```python
from build123d import *

# Parameters (mm, degrees)
SKETCH_W          = 64.5
SKETCH_H          = 46.5
PAD_DEPTH         = 25
SKETCH001_W       = 61
SKETCH001_H       = 42.5
POCKET_DEPTH      = 21
SKETCH002_R       = 2
POCKET001_DEPTH   = 4
POCKET002_DEPTH   = 2
POCKET003_DEPTH   = 2
SKETCH005_R       = 2
POCKET004_DEPTH   = 2
PAD001_DEPTH      = 10
PAD001_DEPTH_BACK = 2
PAD002_DEPTH      = 1
SKETCH008_R       = 5.5
PAD003_DEPTH      = 4
SKETCH009_W       = 5
SKETCH009_H       = 5
POCKET005_DEPTH   = 49.501
SKETCH010_W       = 5
SKETCH010_H       = 5
POCKET006_DEPTH   = 26.7259364864
SKETCH011_W       = 3
SKETCH011_H       = 6
SKETCH011_H_2     = 4
PAD004_DEPTH      = 2
POCKET007_DEPTH   = 5


with BuildPart() as part:
    # Sketch → Pad (new body)
    with BuildSketch(Plane.XZ):
        Rectangle(SKETCH_W, SKETCH_H)
    extrude(amount=PAD_DEPTH)

    # Sketch001 (on Face6 of Pad) → Pocket (cut)
    with BuildSketch(Plane.XZ.offset(25)):
        Rectangle(SKETCH001_W, SKETCH001_H)
    extrude(amount=-POCKET_DEPTH, mode=Mode.SUBTRACT)

    # Sketch002 (on Face11 of Pocket) → Pocket001 (cut)
    with BuildSketch(Plane.XZ.offset(4)):
        with Locations((24.5, 16.25)):
            Circle(SKETCH002_R)
    extrude(amount=-POCKET001_DEPTH, mode=Mode.SUBTRACT)

    # Sketch003 (on Face3 of Pocket001) → Pocket002 (cut)
    with BuildSketch(Plane(origin=(32.25, 0, 0), x_dir=(0, 0, 1), z_dir=(1, 0, 0))):
        with BuildLine():
            ThreePointArc((-7.25, 18.5), (-11.25, 14.5), (-7.25, 10.5))
            Line((-7.25, 10.5), (2.75, 10.5))
            ThreePointArc((2.75, 10.5), (6.75, 14.5), (2.75, 18.5))
            Line((-7.25, 18.5), (2.75, 18.5))
        make_face()
    extrude(amount=-POCKET002_DEPTH, mode=Mode.SUBTRACT)

    # Sketch004 (on Face1 of Pocket002) → Pocket003 (cut)
    with BuildSketch(Plane(origin=(0, 0, 23.25), x_dir=(-1, 0, 0), z_dir=(0, 0, 1))):
        with BuildLine():
            ThreePointArc((8.5, 21.5), (1, 14), (8.5, 6.5))
            Line((8.5, 6.5), (15.5, 6.5))
            ThreePointArc((15.5, 6.5), (23, 14), (15.5, 21.5))
            Line((8.5, 21.5), (15.5, 21.5))
        make_face()
    extrude(amount=-POCKET003_DEPTH, mode=Mode.SUBTRACT)

    # Sketch005 (on Face10 of Pocket003) → Pocket004 (cut)
    with BuildSketch(Plane(origin=(0, 0, -23.25), x_dir=(1, 0, 0), z_dir=(0, 0, -1))):
        with Locations((-21.5, 20)):
            Circle(SKETCH005_R)
    extrude(amount=-POCKET004_DEPTH, mode=Mode.SUBTRACT)

    # Sketch006 (on DatumPlane) → Pad001 (join, two sides)
    with BuildSketch(Plane(origin=(32.25, 0, -23.25), x_dir=(0, 0.9925461516, 0.1218693434), z_dir=(0, 0.1218693434, -0.9925461516))) as pad001_sk:
        with BuildLine():
            Line((0, -15), (0, -49.5))
            Line((0, -49.5), (-7, -49.5))
            ThreePointArc((-7, -15), (-24.25, -32.25), (-7, -49.5))
            Line((0, -15), (-7, -15))
        make_face()
    extrude(amount=PAD001_DEPTH)
    extrude(pad001_sk.sketch, amount=-PAD001_DEPTH_BACK)

    # Sketch007 (on Face10 of Pad001) → Pad002 (join)
    with BuildSketch(Plane(origin=(0, 0, -23.25), x_dir=(1, 0, 0), z_dir=(0, 0, -1))):
        with BuildLine():
            ThreePointArc((14.5355662094, 16.4110180962), (0, 24.4043784957), (-14.5355662094, 16.4110180962))
            Line((-14.5355662094, 16.4110180962), (14.5355662094, 16.4110180962))
        make_face()
    extrude(amount=PAD002_DEPTH)

    # Sketch008 (on Face26 of Pad002) → Pad003 (join)
    with BuildSketch(Plane(origin=(0, 4.0310354704, -32.8301493344), x_dir=(1, 0, 0), z_dir=(0, 0.1218693434, -0.9925461516))):
        with Locations((0, 12)):
            Circle(SKETCH008_R)
    extrude(amount=PAD003_DEPTH)

    # Sketch009 (on Face21 of Pad003) → Pocket005 (cut, through all)
    with BuildSketch(Plane(origin=(17.25, 0, 0), x_dir=(0, 0, 1), z_dir=(1, 0, 0))):
        with Locations((-28.5, 8.5)):
            Rectangle(SKETCH009_W, SKETCH009_H)
    extrude(amount=-POCKET005_DEPTH, mode=Mode.SUBTRACT)

    # Sketch010 (on Face11 of Pocket005) → Pocket006 (cut, through all)
    with BuildSketch(Plane(origin=(0, -2.8123420363, -0.345312182), x_dir=(1, 0, 0), z_dir=(0, 0.9925461516, 0.1218693434))):
        with Locations((0, 27.5)):
            Rectangle(SKETCH010_W, SKETCH010_H)
    extrude(amount=-POCKET006_DEPTH, mode=Mode.SUBTRACT)

    # Sketch011 (on Face1 of Pocket006) → Pad004 (join)
    with BuildSketch(Plane(origin=(0, 0, 23.25), x_dir=(-1, 0, 0), z_dir=(0, 0, 1))):
        with Locations((-4, 3)):
            Rectangle(SKETCH011_W, SKETCH011_H)
        with Locations((4, 3)):
            Rectangle(SKETCH011_W, SKETCH011_H)
        with Locations((-4, 23)):
            Rectangle(SKETCH011_W, SKETCH011_H_2)
        with Locations((4, 23)):
            Rectangle(SKETCH011_W, SKETCH011_H_2)
    extrude(amount=PAD004_DEPTH)

    # Sketch012 (on Face2 of Pad004) → Pocket007 (cut)
    with BuildSketch(Plane(origin=(0, 0, 0), x_dir=(1, 0, 0), z_dir=(0, 1, 0))):
        with BuildLine():
            ThreePointArc((7.5, 4), (0, 11.5), (-7.5, 4))
            Line((-7.5, 4), (-7.5, -4))
            ThreePointArc((-7.5, -4), (0, -11.5), (7.5, -4))
            Line((7.5, 4), (7.5, -4))
        make_face()
    extrude(amount=-POCKET007_DEPTH, mode=Mode.SUBTRACT)


solid = part.part
```
Model file for the job. Use its own axes, mm. A direction names the side the tool comes from. Round coordinates to 2 decimals unless told otherwise and drop trailing zeros. Write each loop counter-clockwise with the first axis right and the second up, starting at its lowest first coordinate (ties: lowest second). Pieces come first, ordered by that corner, then holes. Notation, with made-up numbers: (-27, 5) - (23, 5) arc R16 cw to (23, 19) - close; hole circle Ø9 at (72, -39). An arc over 180 degrees is marked (long way). Use CSV: the item, a comma, the result in double quotes. Start each with the question number.
Item 1: Band-saw the part on C-C (x = -21.5). Write the cut outline in (y, z).
Item 2: Drill centre lines: L1, parallel to X at y = -0.5, z = -3; L2, parallel to Z at x = 25, y = -9; L3, parallel to X at y = -20, z = -21.65. Where is each one in solid material? Low to high. Write a range as [from, to].
Item 3: Band-saw the part on D-D (y = -14.5). State how many separate pieces and enclosed holes the cut face has, and give its area (3 significant figures).
Item 4: Band-saw the part on A-A (z = 16.25). Write the cut outline in (x, y).
Item 5: Band-saw the part on B-B (x = -13.5). Write the cut outline in (y, z).
Item 6: Two-plate mould, pull along Y, no slides. Class faces 4 (the face through (5.5, -3, 24)), 5 (the face through (-8, 0, 1)), 6 (the face through (6, -4, -9)), 7 (the face through (-12, -21.5, 22)): released by +Y, released by -Y, zero draft, split by the parting line, or undercut.
Item 7: Pin check, flat tips, straight feed: P1, Ø6, axis at x = 5, y = -12, coming from the +Z side; P2, Ø2, axis at x = 14.5, z = 16.5, coming from the -Y side; P3, Ø2, axis at y = -3.5, z = 24.5, coming from the +X side. Stop position of each tip, or through.
Item 8: Tool access for faces 1 (the face through (17.25, -3, -28)), 2 (the face through (2.5, -23, 24)), 3 (the face through (0.2, -11, -26.3)): list every direction of +Z, -Z, +X, -X, +Y, -Y with a clear straight run to the whole face (end or side of a thin tool).
Checked values:
1,outline,"(-25, -23.25) - (-22, -23.25) - (-22, -21.25) - (-25, -21.25) - close; (-25, 21.25) - (-18.5, 21.25) - (-18.5, 23.25) - (-25, 23.25) - close; (-18, -23.25) - (0, -23.25) - (0, 23.25) - (-9.5, 23.25) - (-9.5, 21.25) - (-4, 21.25) - (-4, -21.25) - (-18, -21.25) - close"
2,L1,"x = [-32.25, -7.5], [7.5, 32.25]"
2,L2,"z = [-23.25, -21.25], [21.25, 23.25]"
2,L3,"x = [-32.25, -23.5], [-19.5, 32.25]"
3,separate pieces,"2"
3,enclosed holes,"1"
3,area,"667 mm²"
4,outline,"(-32.25, -25) - (-30.5, -25) - (-30.5, -4) - (22.5, -4) - (22.5, 0) - (-32.25, 0) - close; (26.5, -4) - (30.5, -4) - (30.5, -25) - (32.25, -25) - (32.25, 0) - (26.5, 0) - close"
5,outline,"(-25, -23.25) - (-17.87, -23.25) - (-17.87, -24.25) - (-17.75, -24.25) - (-16.39, -35.34) - (1.22, -33.18) - (0, -23.25) - (0, 23.25) - (-6.5, 23.25) - (-6.5, 21.25) - (-4, 21.25) - (-4, -21.25) - (-25, -21.25) - close; (-25, 21.25) - (-21.5, 21.25) - (-21.5, 23.25) - (-25, 23.25) - close; hole (-11, -31) - (-6, -31) - (-6, -26) - (-11, -26) - close"
6,face 4,"zero draft"
6,face 5,"released by +Y"
6,face 6,"released by -Y"
6,face 7,"undercut"
7,P1,"stops at z = 23.25"
7,P2,"stops at y = -4"
7,P3,"stops at x = 5.5"
8,face 1,"-Z, +X, +Y, -Y"
8,face 2,"+Z, +Y, -Y"
8,face 3,"+X, -X"
